Read the model definition and answer for the solid it produces. Units are mm, in the model's axes. A direction names the side the tool comes from. Round coordinates to 2 decimals unless told otherwise and drop trailing zeros. Loops run counter-clockwise (first coordinate to the right, second up) from the corner with the lowest first, then second, coordinate; pieces in that order, holes last. Notation, with made-up numbers: M -20,39.5 L 36,39.5 A15 ccw 36,46.5 Z; hole C 3.5,-37 d1. An arc over 180 degrees is marked long. Answer as CSV lines item,"result".
```python
from build123d import *

# Parameters (mm, degrees)
F0_W     = 139.96376
F0_H     = 89.45696
F1_DEPTH = 54
F3_W     = 119.418622
F3_H     = 92.025094
F4_DEPTH = 98
F5_W     = 77.472278
F5_H     = 29.961662
F6_DEPTH = 195
F7_R     = 13.686729
F8_DEPTH = 202


with BuildPart() as f1:
    # F0 (on Front) → F1 (new body)
    with BuildSketch(Plane.XZ):
        Rectangle(F0_W, F0_H)
    extrude(amount=F1_DEPTH)

    # F2: F1 across face


with BuildPart() as f1_1:
    add(f1.part)
    add(f1.part.mirror(Plane(origin=(0, 0, 0), x_dir=(1, 0, 0), z_dir=(0, 1, 0))))

    # F3 (on face) → F4 (cut)
    with BuildSketch(Plane.XY.offset(44.72848)):
        Rectangle(F3_W, F3_H)
    extrude(amount=-F4_DEPTH, mode=Mode.SUBTRACT)

    # F5 (on face) → F6 (cut)
    with BuildSketch(Plane.XZ.offset(54)):
        with Locations((1e-06, 29.747649)):
            Rectangle(F5_W, F5_H)
    extrude(amount=-F6_DEPTH, mode=Mode.SUBTRACT)

    # F7 (on face) → F8 (cut)
    with BuildSketch(Plane(origin=(-69.98188, 0, 0), x_dir=(0, -1, 0), z_dir=(-1, 0, 0))):
        Circle(F7_R)
    extrude(amount=-F8_DEPTH, mode=Mode.SUBTRACT)


solid = f1_1.part
```
1) Determine the mould class of faces 1 (the flat face through (-1, -46.013, -9)), 2 (the flat face through (-1, -54, -9)), 3 (the flat face through (-62, -1, 44.728)) for opening direction Y: released by +Y, released by -Y, zero draft, split by the parting line, or undercut.
Evaluation:
face 1,"undercut"
face 2,"released by -Y"
face 3,"zero draft"
2) Find section C-C, the plane y = 33. Give the vertices of the cut face in (x, z), then the cut area to 3 significant figures.
Evaluation:
outline,"M -69.98,-44.73 L -59.71,-44.73 L -59.71,44.73 L -69.98,44.73 Z; M 59.71,-44.73 L 69.98,-44.73 L 69.98,44.73 L 59.71,44.73 Z"
area,"1,840 mm^2"
3) Find section D-D, the plane y = 0. Give the vertices of the cut face in (x, z).
Evaluation:
outline,"M -69.98,-44.73 L -59.71,-44.73 L -59.71,-13.69 L -69.98,-13.69 Z; M -69.98,13.69 L -59.71,13.69 L -59.71,44.73 L -69.98,44.73 Z; M 59.71,-44.73 L 69.98,-44.73 L 69.98,-13.69 L 59.71,-13.69 Z; M 59.71,13.69 L 69.98,13.69 L 69.98,44.73 L 59.71,44.73 Z"
4) Find section B-B, the plane x = -55. Give the vertices of the cut face in (y, z), then the cut area to 3 significant figures.
Evaluation:
outline,"M -54,-44.73 L -46.01,-44.73 L -46.01,44.73 L -54,44.73 Z; M 46.01,-44.73 L 54,-44.73 L 54,44.73 L 46.01,44.73 Z"
area,"1,430 mm^2"
5) Find section A-A, the plane z = 35. Give the vertices of the cut face in (x, y), then the cut area to 3 significant figures.
Evaluation:
outline,"M -69.98,-54 L -38.74,-54 L -38.74,-46.01 L -59.71,-46.01 L -59.71,46.01 L -38.74,46.01 L -38.74,54 L -69.98,54 Z; M 38.74,-54 L 69.98,-54 L 69.98,54 L 38.74,54 L 38.74,46.01 L 59.71,46.01 L 59.71,-46.01 L 38.74,-46.01 Z"
area,"2,890 mm^2"
6) This flat-tipped pin is pushed along its axis until it touches: P1, Ø9, axis at x = -2, y = 51.5, coming from the +Z side. Where does it stop, or does it pass through?
Evaluation:
P1,"stops at z = 14.77"
7) Straight lines are drawn through the part: line 1 (Y direction, x = 53.5, z = 28.5); line 2 (X direction, y = -8, z = 25); line 3 (Z direction, x = 63.5, y = 0). For each, find the intervals that lie inside material, in ascending order.
Evaluation:
line 1,"y = -54 to -46.01, 46.01 to 54"
line 2,"x = -69.98 to -59.71, 59.71 to 69.98"
line 3,"z = -44.73 to -13.69, 13.69 to 44.73"
8) A tool of negligible diameter and unlimited length cuts with its end or side. For faces 4 (the flat face through (-59.709, -11, 11)), 5 (the flat face through (38.736, 50, 30)), 6 (the cylindrical face through (-64.918, -13.055, 4.111)), from which of +Z, -Z, +X, -X, +Y, -Y can it reach the whole face along a straight path? Write none if from no direction.
Evaluation:
face 4,"+Z, -Z"
face 5,"+Z, +Y, -Y"
face 6,"+X, -X"
